Could you check a few things on this model? Use its own coordinates, in mm. A direction names the side the tool comes from. Give positions to 0.01 mm unless a question says otherwise; leave off trailing zeros. Write each loop counter-clockwise with the first axis right and the second up, starting at its lowest first coordinate (ties: lowest second). Pieces come first, ordered by that corner, then holes. Notation, with made-up numbers: (-37.75, 3) - (9.25, 3) arc R24 cw to (9.25, 16) - close; hole circle Ø2 at (-35, 6). An arc over 180 degrees is marked (long way). Answer in a Markdown table with one row per item.
from build123d import *

# Parameters (mm, degrees)
F0_R        = 3.81
F1_DEPTH    = 1.016
F2_W        = 4.2779184878
F2_H        = 13.4340701625
F3_DEPTH    = 1.016
F4_SIZE     = 2.286
F5_T1_DEPTH = 11.4673196631


# Not quite as in the source:
# - a fillet or chamfer that OpenCascade refuses, or shapes differently, is made with other operations: its cross-section is extruded or revolved along the edge and cut away or added


with BuildPart() as f1:
    # F0 (on Top) → F1 (new body)
    with BuildSketch(Plane.XY):
        with Locations((-29.276387766, 26.0032489896)):
            Circle(F0_R)
    extrude(amount=F1_DEPTH)

    # F2 (on Top) → F3 (join)
    with BuildSketch(Plane.XY):
        with Locations((-29.5591074973, 16.392851714)):
            Rectangle(F2_W, F2_H)
    extrude(amount=F3_DEPTH)

    # F4
    f4_edges = [f1.edges().sort_by_distance(p)[0] for p in [
        (-27.420148, 9.675817, 0.508),
    ]]
    chamfer(f4_edges, length=F4_SIZE)

    # F5: chamfer of 2.032 on 1 edges, made by hand

    # F5_s2 → F5_t1 (cut)
    with BuildSketch(Plane.XY.offset(-5.2256598315)):
        Polygon((-29.6660667412, 9.6758166328), (-31.6980667412, 11.7078166328), (-31.6980667412, 9.6758166328), align=None)
    extrude(amount=F5_T1_DEPTH, mode=Mode.SUBTRACT)


solid = f1.part
1) If I drill on line 1 (X direction, y = 21.75, z = 0.1); line 2 (Y direction, x = -26, z = 0.3); line 3 (Y direction, x = -29.75, z = 0.55), over which ranges is the centre line in solid material (lowest first)?
Check values:
| item | result |
|---|---|
| line 1 | x = -31.7 to -27.42 |
| line 2 | y = 24.06 to 27.95 |
| line 3 | y = 9.76 to 29.78 |
2) On a 3-axis mill with a long thin cutter (end or side, diameter ignored), from which of +Z, -Z, +X, -X, +Y, -Y can I reach the whole of each face in a straight line? I mean faces 1 (the face through (-31.698, 17.3, 0.5)), 2 (the face through (-27.42, 17.2, 0.5)), 3 (the face through (-29, 22, 1.016)). Say none if no direction works.
Check values:
| item | result |
|---|---|
| face 1 | +Z, -Z, -X, -Y |
| face 2 | +Z, -Z, +X, -Y |
| face 3 | +Z, +X, -X, +Y, -Y |
3) Imagine slicing it at C-C (x = -31.5). List the corners of the cut face in (y, z) for me, then the cut area to 3 significant figures.
Check values:
| item | result |
|---|---|
| outline | (11.51, 0) - (29.1, 0) - (29.1, 1.02) - (11.51, 1.02) - close |
| area | 17.9 mm2 |
4) Imagine slicing it at A-A (z = 0.7). List the corners of the cut face in (x, y) for me.
Check values:
| item | result |
|---|---|
| outline | (-31.7, 11.71) - (-29.69, 9.7) - (-27.42, 11.96) - (-27.42, 22.68) arc R3.81 ccw (long way) to (-31.7, 23.06) - close |
5) Imagine slicing it at B-B (y = 13.5). List the corners of the cut face in (x, z) for me.
Check values:
| item | result |
|---|---|
| outline | (-31.7, 0) - (-27.42, 0) - (-27.42, 1.02) - (-31.7, 1.02) - close |
